Geometry: final body of the model. Coordinates: model frame, mm. Face numbers are marked on the shaded views. A direction names the side the tool comes from. Give positions to 0.01 mm unless a question says otherwise; leave off trailing zeros. Loops run counter-clockwise (first coordinate to the right, second up) from the corner with the lowest first, then second, coordinate; pieces in that order, holes last. Notation, with made-up numbers: M 70.5,18 L 125.5,18 A21 ccw 125.5,38 Z; hole C 41.25,11 d9. An arc over 180 degrees is marked long. Put each result on its own line as item: value.
```python
from build123d import *

# Parameters (mm, degrees)
SKETCH1_W               = 125
SKETCH1_H               = 20
BOSS_EXTRUDE1_DEPTH     = 100
SKETCH8_W               = 20
SKETCH8_H               = 20
BOSS_EXTRUDE2_DEPTH     = 20
SKETCH11_R              = 4.05
CUT_EXTRUDE3_DEPTH      = 40
SKETCH9_W               = 20
SKETCH9_H               = 20
BOSS_EXTRUDE3_DEPTH     = 20
SKETCH10_R              = 2
CUT_EXTRUDE2_DEPTH      = 20
ESQUISSE2_W             = 165
ESQUISSE2_H             = 1.05
ENL_V_MAT_EXTRU_1_DEPTH = 10


with BuildPart() as part:
    # Sketch1 → Boss-Extrude1 (new body)
    with BuildSketch(Plane.XY):
        with Locations((62.5, 10)):
            Rectangle(SKETCH1_W, SKETCH1_H)
    extrude(amount=BOSS_EXTRUDE1_DEPTH)

    # Sketch8 → Boss-Extrude2 (add)
    with BuildSketch(Plane.ZY):
        with Locations((90, 10)):
            Rectangle(SKETCH8_W, SKETCH8_H)
    extrude(amount=BOSS_EXTRUDE2_DEPTH)

    # Sketch11 → Cut-Extrude3 (cut)
    with BuildSketch(Plane(origin=(0, 20, 0), x_dir=(1, 0, 0), z_dir=(0, 1, 0))):
        with Locations(Location((22.5, -35, 0), (0, 0, 270))):
            Circle(SKETCH11_R)
        with Locations(Location((22.5, -65, 0), (0, 0, 270))):
            Circle(SKETCH11_R)
        with Locations(Location((102.5, -65, 0), (0, 0, 270))):
            Circle(SKETCH11_R)
        with Locations(Location((102.5, -35, 0), (0, 0, 270))):
            Circle(SKETCH11_R)
    extrude(amount=-CUT_EXTRUDE3_DEPTH, mode=Mode.SUBTRACT)

    # Sketch9 → Boss-Extrude3 (add)
    with BuildSketch(Plane(origin=(125, 0, 0), x_dir=(0, 0, -1), z_dir=(1, 0, 0))):
        with Locations((-90, 10)):
            Rectangle(SKETCH9_W, SKETCH9_H)
    extrude(amount=BOSS_EXTRUDE3_DEPTH)

    # Sketch10 → Cut-Extrude2 (cut)
    with BuildSketch(Plane(origin=(0, 0, 80), x_dir=(-1, 0, 0), z_dir=(0, 0, -1))):
        with Locations((10, 5)):
            Circle(SKETCH10_R)
        with Locations(Location((-135, 5, 0), (0, 0, 180))):
            Circle(SKETCH10_R)
    extrude(amount=-CUT_EXTRUDE2_DEPTH, mode=Mode.SUBTRACT)

    # Esquisse2 → Enlèv. mat.-Extru.1 (cut)
    with BuildSketch(Plane(origin=(0, 20, 0), x_dir=(1, 0, 0), z_dir=(0, 1, 0))):
        with Locations((62.5, -99.475)):
            Rectangle(ESQUISSE2_W, ESQUISSE2_H)
    extrude(amount=-ENL_V_MAT_EXTRU_1_DEPTH, mode=Mode.SUBTRACT)


solid = part.part
```
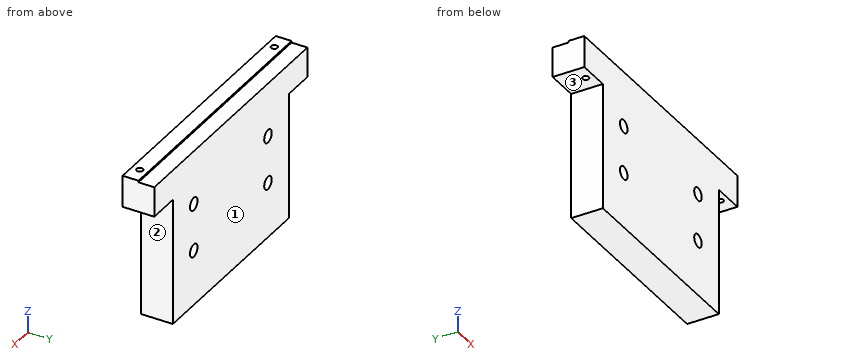
Item 1: Section D-D on y = 12.5. Output: boundary loops of the cut face in (x, z).
Output values:
outline: M -20,80 L 0,80 L 0,0 L 125,0 L 125,80 L 145,80 L 145,98.95 L -20,98.95 Z; hole C 22.5,35 d8.1; hole C 22.5,65 d8.1; hole C 102.5,35 d8.1; hole C 102.5,65 d8.1
Item 2: Section C-C on x = 135. Output: boundary loops of the cut face in (y, z), then the cut area to 4 significant figures.
Output values:
outline: M 0,80 L 3,80 L 3,100 L 0,100 Z; M 7,80 L 20,80 L 20,98.95 L 10,98.95 L 10,100 L 7,100 Z
area: 309.5 mm²
Item 3: Section A-A on y = 5. Output: boundary loops of the cut face in (x, z).
Output values:
outline: M -20,80 L -12,80 L -12,100 L -20,100 Z; M -8,80 L 0,80 L 0,0 L 125,0 L 125,80 L 133,80 L 133,100 L -8,100 Z; M 137,80 L 145,80 L 145,100 L 137,100 Z; hole C 22.5,35 d8.1; hole C 22.5,65 d8.1; hole C 102.5,35 d8.1; hole C 102.5,65 d8.1
Item 4: Pin query (flat end, axial travel): pin 1 Ø10 at (x, y) = (131, 12.5) entering from -Z; pin 2 Ø5 at (y, z) = (17.5, 61.5) entering from +X; pin 3 Ø6 at (y, z) = (3.5, 57.5) entering from -X. Return the tip coordinate at first contact, or that it passes through.
Output values:
pin 1: z = 80
pin 2: x = 125
pin 3: x = 0
Item 5: Line query: probe 1 along X at (y, z) = (11.25, 35); probe 2 along X at (y, z) = (9.25, 64); probe 3 along Y at (x, z) = (-10, 93.75). Output: solid intervals per line, ascending. Write a range as [from, to].
Output values:
probe 1: [0, 18.45], [26.55, 98.45], [106.55, 125]
probe 2: [0, 18.58], [26.42, 98.58], [106.42, 125]
probe 3: [0, 3], [7, 20]
Item 6: Set-up query: the marked faces 1, 2 and 3. Return all of +Z, -Z, +X, -X, +Y, -Y with unobstructed straight access to the full face (end or side cutting, diameter ignored); none if empty.
Output values:
face 1: +Z, -Z, +X, -X, +Y
face 2: -Z, +X, +Y, -Y
face 3: -Z, -X, +Y, -Y
Item 7: Section B-B on z = 35. Output: boundary loops of the cut face in (x, y).
Output values:
outline: M 0,0 L 18.45,0 L 18.45,20 L 0,20 Z; M 26.55,0 L 98.45,0 L 98.45,20 L 26.55,20 Z; M 106.55,0 L 125,0 L 125,20 L 106.55,20 Z
